```python
from build123d import *
from build123d.topology import SkipClean

# Parameters (mm, degrees)
IZIM1_R                     = 3.5
Y_KSEKLIK_EKSTR_ZYON1_DEPTH = 40
KES_EKSTR_ZYON1_DEPTH       = 46.058295574
KES_EKSTR_ZYON1_DEPTH_BACK  = 46.058295574
IZIM3_W                     = 10
IZIM3_H                     = 10
KES_EKSTR_ZYON2_DEPTH       = 46.771852704
IZIM5_R                     = 2.5
KES_EKSTR_ZYON4_DEPTH       = 46
PAH1_SIZE                   = 3
IZIM4_W                     = 0.5
IZIM4_H                     = 10
KES_EKSTR_ZYON5_DEPTH       = 46
PAH2_SIZE                   = 2
BOSS_EXTRUDE1_START         = -10
SKETCH1_R                   = 3.5
BOSS_EXTRUDE1_DEPTH         = 10
BOSS_EXTRUDE2_START         = -10
SKETCH2_R                   = 3.5
BOSS_EXTRUDE2_DEPTH         = 10
CUT_EXTRUDE1_DEPTH          = 0.2
CUT_EXTRUDE2_DEPTH          = 0.2
CUT_EXTRUDE3_START          = -0.1
CUT_EXTRUDE3_DEPTH          = 0.1


with BuildPart() as part:
    # Çizim1 → Yükseklik-Ekstrüzyon1 (new body)
    with BuildSketch(Plane.XY):
        with BuildLine():
            Line((0, 5), (5, 5))
            Line((5, 5), (5, 5.5))
            Line((5, 5.5), (20, 5.5))
            Line((20, 5.5), (20, 5))
            Line((20, 5), (20, 0.5))
            Line((20, 0.5), (4.974937186, 0.5))
            ThreePointArc((4.974937186, 0.5), (-3.354101966, -3.708099244), (0, 5))
        make_face()
        Circle(IZIM1_R, mode=Mode.SUBTRACT)
    extrude(amount=Y_KSEKLIK_EKSTR_ZYON1_DEPTH)

    # Çizim2 → Kes-Ekstrüzyon1 (cut, two sides: drawn at the far end of the back side and taken through both)
    with BuildSketch(Plane.XY.offset(40).offset(-KES_EKSTR_ZYON1_DEPTH_BACK)):
        Polygon((-72.503925857, -4.25), (-6.336762511, -4.25), (12.42239056, -4.25), (78.589553905, -4.25), (78.589553905, -136.584326691), (-72.503925857, -136.584326691), align=None)
    extrude(amount=KES_EKSTR_ZYON1_DEPTH + KES_EKSTR_ZYON1_DEPTH_BACK, mode=Mode.SUBTRACT)

    # Çizim3 → Kes-Ekstrüzyon2 (cut, through all)
    with BuildSketch(Plane.XZ.offset(4.25)):
        with Locations((0, 25)):
            Rectangle(IZIM3_W, IZIM3_H)
        with Locations((0, 5)):
            Rectangle(IZIM3_W, IZIM3_H)
    extrude(amount=-KES_EKSTR_ZYON2_DEPTH, mode=Mode.SUBTRACT)

    # Çizim5 → Kes-Ekstrüzyon4 (cut, through all)
    with BuildSketch(Plane.XZ.offset(-0.5)):
        with Locations(Location((12.5, 7.5, 0), (0, 0, 270))):
            Circle(IZIM5_R)
        with Locations(Location((12.5, 32.5, 0), (0, 0, 90))):
            Circle(IZIM5_R)
    extrude(amount=-KES_EKSTR_ZYON4_DEPTH, mode=Mode.SUBTRACT)

    # Pah1
    pah1_edges = [part.edges().sort_by_distance(p)[0] for p in [
        (20, 0.5, 20),
        (12.487468593, 0.5, 40),
        (12.5, 0.5, 0),
    ]]
    chamfer(pah1_edges, length=PAH1_SIZE)

    # Çizim4 → Kes-Ekstrüzyon5 (cut, through all)
    with BuildSketch(Plane.XZ.offset(-0.5)):
        with Locations((5.224937186, 25)):
            Rectangle(IZIM4_W, IZIM4_H)
        with Locations((5.25, 5)):
            Rectangle(IZIM4_W, IZIM4_H)
    extrude(amount=-KES_EKSTR_ZYON5_DEPTH, mode=Mode.SUBTRACT)

    # Pah2
    pah2_edges = [part.edges().sort_by_distance(p)[0] for p in [
        (12.5, 0.5, 10),
        (12.5, 0.5, 30),
    ]]
    chamfer(pah2_edges, length=PAH2_SIZE - 0.0001)  # a hair under: the kernel refuses the full size

    # Sketch1 → Boss-Extrude1 (add)
    with BuildSketch(Plane.XY.offset(40).offset(BOSS_EXTRUDE1_START)):
        with Locations(Location((0, 0, 0), (0, 0, 180))):
            Circle(SKETCH1_R)
    extrude(amount=BOSS_EXTRUDE1_DEPTH)

    # Sketch2 → Boss-Extrude2 (add)
    with BuildSketch(Plane.XY.offset(20).offset(BOSS_EXTRUDE2_START)):
        Circle(SKETCH2_R)
    extrude(amount=BOSS_EXTRUDE2_DEPTH)

    # Sketch3 → Cut-Extrude1 (cut)
    with BuildSketch(Plane(origin=(0, 0, 30), x_dir=(-1, 0, 0), z_dir=(0, 0, -1))):
        with BuildLine():
            Line((0, 5), (-5, 5))
            Line((-5, 5), (-5, 5.5))
            Line((-5, 5.5), (-5.474937186, 5.5))
            Line((-5.474937186, 5.5), (-5.474937186, 0.5))
            Line((-5.474937186, 0.5), (-4.974937186, 0.5))
            ThreePointArc((-4.974937186, 0.5), (-4.484894308, -2.210367175), (-2.633913438, -4.25))
            Line((-2.633913438, -4.25), (2.633913438, -4.25))
            ThreePointArc((2.633913438, -4.25), (4.808846015, 1.369306394), (0, 5))
        make_face()
    extrude(amount=-CUT_EXTRUDE1_DEPTH, mode=Mode.SUBTRACT)

    # Sketch4 → Cut-Extrude2 (cut)
    with BuildSketch(Plane(origin=(0, 0, 10), x_dir=(-1, 0, 0), z_dir=(0, 0, -1))):
        with BuildLine():
            Line((-2.633913438, -4.25), (2.633913438, -4.25))
            ThreePointArc((2.633913438, -4.25), (4.808846015, 1.369306394), (0, 5))
            Line((0, 5), (-5, 5))
            Line((-5, 5), (-5, 5.5))
            Line((-5, 5.5), (-5.5, 5.5))
            Line((-5.5, 5.5), (-5.5, 0.5))
            Line((-5.5, 0.5), (-4.974937186, 0.5))
            ThreePointArc((-4.974937186, 0.5), (-4.484894308, -2.210367175), (-2.633913438, -4.25))
        make_face()
    extrude(amount=-CUT_EXTRUDE2_DEPTH, mode=Mode.SUBTRACT)

    # Sketch5 → Cut-Extrude3 (cut)
    with BuildSketch(Plane.XY.offset(20).offset(CUT_EXTRUDE3_START)):
        with BuildLine():
            Line((4.974937186, 0.5), (5.474937186, 0.5))
            Line((5.474937186, 0.5), (5.474937186, 5.5))
            Line((5.474937186, 5.5), (5, 5.5))
            Line((5, 5.5), (5, 5))
            Line((5, 5), (0, 5))
            ThreePointArc((0, 5), (-4.808846015, 1.369306394), (-2.633913438, -4.25))
            Line((-2.633913438, -4.25), (2.633913438, -4.25))
            ThreePointArc((2.633913438, -4.25), (4.484894308, -2.210367175), (4.974937186, 0.5))
        make_face()
    extrude(amount=CUT_EXTRUDE3_DEPTH, mode=Mode.SUBTRACT)

    # Sketch6 → Revolve1 (revolve)
    with BuildSketch(Plane(origin=(0, 0.375, 0), x_dir=(-1, 0, 0), z_dir=(0, -1, 0)), mode=Mode.PRIVATE) as revolve1_sk:
        with BuildLine():
            ThreePointArc((0, -7.2), (-3, -10.2), (0, -13.2))
            Line((0, -13.2), (0, -7.2))
        make_face()
        with BuildLine():
            Line((0, -7.2), (0, -13.2))
            ThreePointArc((0, -13.2), (2.121320344, -12.321320344), (3, -10.2))
            ThreePointArc((3, -10.2), (2.121320344, -8.078679656), (0, -7.2))
        make_face()
    revolve(revolve1_sk.sketch.rotate(Axis((0, 0.375, 13.2), (0, 0, -1)), 180), axis=Axis((0, 0.375, 13.2), (0, 0, -1)))

    # Sketch6<7> → Cut-Revolve1 (revolve, cut)
    with SkipClean():  # the faces are left unmerged after this step: merging them gives an invalid solid
        with BuildSketch(Plane(origin=(0, 0.375, 0), x_dir=(-1, 0, 0), z_dir=(0, -1, 0)), mode=Mode.PRIVATE) as cut_revolve1_sk:
            with BuildLine():
                ThreePointArc((0, -27.2), (-3, -30.2), (0, -33.2))
                Line((0, -33.2), (0, -27.2))
            make_face()
            with BuildLine():
                Line((0, -27.2), (0, -33.2))
                ThreePointArc((0, -33.2), (2.121320344, -32.321320344), (3, -30.2))
                ThreePointArc((3, -30.2), (2.121320344, -28.078679656), (0, -27.2))
            make_face()
        revolve(cut_revolve1_sk.sketch.rotate(Axis((0, 0.375, 33.2), (0, 0, -1)), 180), axis=Axis((0, 0.375, 33.2), (0, 0, -1)), mode=Mode.SUBTRACT)
    add(part.part.scale(1), mode=Mode.REPLACE)  # the faces are merged on a copy


solid = part.part
```
Work out the finished part from the listing and answer in its coordinate system (mm). A direction names the side the tool comes from. Give positions to 0.01 mm unless a question says otherwise; leave off trailing zeros. Loops run counter-clockwise (first coordinate to the right, second up) from the corner with the lowest first, then second, coordinate; pieces in that order, holes last. Notation, with made-up numbers: M 25,-16.5 L 62,-16.5 A21 ccw 62,-12.5 Z; hole C 9.5,84 d6. An arc over 180 degrees is marked long. One line per item, written item: value. Start each with the question number.
1. Find section C-C (y = -1). Give the vertices of the cut face in (x, z).
2. Find the intervals of material crossed by probe 1 along X at (y, z) = (4.4, 7.5); probe 2 along Z at (x, y) = (12.25, 3.75); probe 3 along Z at (x, y) = (-2, -3.75), in increasing order.
3. Find section A-A (x = 12.5). State how many separate pieces and enclosed holes the cut face has, and give its area (3 significant figures).
4. Each of these flat-tipped pins is pushed along its axis until it touches: P1, Ø3.5, axis at x = 9.5, z = 26, coming from the -Y side; P2, Ø5.5, axis at x = 1.5, z = 13.5, coming from the +Y side; P3, Ø8, axis at x = 12.5, z = 32.5, coming from the -Y side. Where does it stop, or does it pass through?
5. Find section D-D (y = 4.25). Give the vertices of the cut face in (x, z).
6. Which of the six approach directions +Z, -Z, +X, -X, +Y, -Y give full straight-line access (tool end or side, diameter ignored) to faces 5 (the face through (0, 1, 19.9)), 6 (the face through (3, 2, 10.2)), 7 (the face through (2, 5, 35)), 8 (the face through (2, 2, 40))?
7. Determine the mould class of faces 1 (the face through (20, 5, 20)), 2 (the face through (3, -1, 30.2)), 3 (the face through (14.94, 3.98, 31.96)), 4 (the face through (5.5, 3, 5)) for opening direction X: released by +X, released by -X, zero draft, split by the parting line, or undercut.
Reported:
1. outline: M -4.9,10.2 L -2.67,10.2 A2.67 ccw 2.67,10.2 L 4.9,10.2 L 4.9,19.9 L -4.9,19.9 Z; M -4.9,30.2 L -2.67,30.2 A2.67 cw 2.67,30.2 L 4.9,30.2 L 4.9,40 L -4.9,40 Z
2. probe 1: x = 5.5 to 10, 15 to 20
2. probe 2: z = 0 to 5.01, 9.99 to 30.01, 34.99 to 40
2. probe 3: z = 10.2 to 19.9, 30.2 to 40
3. separate pieces: 3
3. enclosed holes: 0
3. area: 133 mm²
4. P1: stops at y = 0.5
4. P2: stops at y = 5
4. P3: stops at y = 1
5. outline: M -2.63,10.2 L 5.5,10.2 L 5.5,0 L 20,0 L 20,40 L -2.63,40 L -2.63,30.2 L 5.47,30.2 L 5.47,19.9 L -2.63,19.9 Z; hole C 12.5,7.5 d5; hole C 12.5,32.5 d5
6. face 5: -X, +Y, -Y
6. face 6: -Z
6. face 7: +Z, -Z, -X, +Y
6. face 8: +Z, +X, -X, +Y, -Y
7. face 1: released by +X
7. face 2: zero draft
7. face 3: undercut
7. face 4: undercut
